CAD build for the part. Positions are in the model's coordinates, mm. Face numbers are marked on the shaded views. A direction names the side the tool comes from. Coordinates: 2 decimals unless noted, no trailing zeros. Order: outer loops, then holes, each group sorted by start corner. A loop starts at its lowest first (then second) coordinate and runs counter-clockwise, first axis right, second up. Notation, with made-up numbers: M -33,6.5 L 24,6.5 A28 cw 24,32.5 Z; hole C -34.75,-25.75 d11. An arc over 180 degrees is marked long. One line per item, written item: value.
from build123d import *

# Parameters (mm, degrees)
SKETCH_1_W                = 48.51
SKETCH_1_H                = 34
SKETCH_1_W_2              = 28.51
SKETCH_1_H_2              = 14
EXTRUDE_1_DEPTH           = 12.25
SKETCH_2_R                = 1.91
CUT_EXTRUDE_1_DEPTH       = 33.05257439
SKETCH_4_W                = 13
SKETCH_4_H                = 13.91
EXTRUDE_1_2_DEPTH         = 74.82
SKETCH_5_W                = 13.91
SKETCH_5_H                = 16.23
EXTRUDE_2_DEPTH           = 15
SKETCH_7_R                = 24.5
SKETCH_7_R_2              = 14.5
EXTRUDE_2_2_DEPTH         = 16.23
SKETCH_12_R               = 1.9
CUT_EXTRUDE_4_DEPTH       = 97.312124675
EXTRUDE_3_DEPTH           = 10
EXTRUDE_3_DEPTH_BACK      = 8
SKETCH_13_W               = 13.91
SKETCH_13_H               = 16.23
SKETCH_14_R               = 1.9
CUT_EXTRUDE_5_DEPTH       = 103.744583434
SKETCH_16_W               = 90.709398763
SKETCH_16_H               = 28.955068616
CUT_EXTRUDE_7_DEPTH       = 111.229011154
SKETCH_18_W               = 13
SKETCH_18_H               = 93.080932143
CUT_EXTRUDE_10_DEPTH      = 27
CUT_EXTRUDE_11_DEPTH      = 57
CUT_EXTRUDE_11_DEPTH_BACK = 27
SKETCH_17_W               = 20.23049449
SKETCH_17_H               = 80.723570055
SKETCH_21_W               = 15.09856282
SKETCH_21_H               = 42.5
EXTRUDE_6_DEPTH           = 10
SKETCH_22_R               = 4.005
CUT_EXTRUDE_12_DEPTH      = 24
SKETCH_23_W               = 15.09856282
SKETCH_23_H               = 4.587452919
CUT_EXTRUDE_13_DEPTH      = 85.439664289


with BuildPart() as part:
    # 草圖1 → Extrude 1 (new body)
    with BuildSketch(Plane(origin=(0, 0, 0), x_dir=(1, 0, 0), z_dir=(0, 1, 0))):
        Rectangle(SKETCH_1_W, SKETCH_1_H)
        Rectangle(SKETCH_1_W_2, SKETCH_1_H_2, mode=Mode.SUBTRACT)
    extrude(amount=EXTRUDE_1_DEPTH)

    # 草圖2 → 除料-伸長1 (cut, through all)
    with BuildSketch(Plane(origin=(0, 12.25, 0), x_dir=(1, 0, 0), z_dir=(0, 1, 0))):
        with Locations(Location((-19.255, 0, 0), (0, 0, 270))):
            Circle(SKETCH_2_R)
        with Locations(Location((19.255, 0, 0), (0, 0, 270))):
            Circle(SKETCH_2_R)
    extrude(amount=-CUT_EXTRUDE_1_DEPTH, mode=Mode.SUBTRACT)

    # 草圖4 → Extrude 1 2 (add)
    with BuildSketch(Plane.XZ):
        with Locations((17.755, 0)):
            Rectangle(SKETCH_4_W, SKETCH_4_H)
    extrude(amount=EXTRUDE_1_2_DEPTH)

    # 草圖5 → Extrude 2 (add)
    with BuildSketch(Plane.ZY.offset(-11.255)):
        with Locations((0, -66.705)):
            Rectangle(SKETCH_5_W, SKETCH_5_H)
    extrude(amount=EXTRUDE_2_DEPTH)

    # 草圖7 → Extrude 2 2 (add)
    with BuildSketch(Plane(origin=(3.626674765, -74.82, 0), x_dir=(1, 0, 0), z_dir=(0, -1, 0))):
        with Locations((-30.978154344, 0)):
            Circle(SKETCH_7_R)
        with Locations((-30.978154344, 0)):
            Circle(SKETCH_7_R_2, mode=Mode.SUBTRACT)
    extrude(amount=-EXTRUDE_2_2_DEPTH)

    # 草圖12 → 除料-伸長4 (cut, through all)
    with BuildSketch(Plane(origin=(0, 0, -6.955), x_dir=(-1, 0, 0), z_dir=(0, 0, -1))):
        with Locations((-3.856713649, -66.705)):
            Circle(SKETCH_12_R)
    extrude(amount=-CUT_EXTRUDE_4_DEPTH, mode=Mode.SUBTRACT)

    # 草圖13 → 填料-伸長3 (add, two sides: drawn at the far end of the back side and taken through both)
    with BuildSketch(Plane(origin=(-55, 0, 0), x_dir=(0, 0, -1), z_dir=(1, 0, 0)).offset(-EXTRUDE_3_DEPTH_BACK)):
        with Locations((0, -66.705)):
            Rectangle(SKETCH_13_W, SKETCH_13_H)
    extrude(amount=EXTRUDE_3_DEPTH + EXTRUDE_3_DEPTH_BACK)

    # 草圖14 → 除料-伸長5 (cut, through all)
    with BuildSketch(Plane(origin=(0, 0, -6.955), x_dir=(-1, 0, 0), z_dir=(0, 0, -1))):
        with Locations((56.908040017, -66.705)):
            Circle(SKETCH_14_R)
    extrude(amount=-CUT_EXTRUDE_5_DEPTH, mode=Mode.SUBTRACT)

    # 草圖16 → 除料-伸長7 (cut, through all)
    with BuildSketch(Plane(origin=(0, 12.25, 0), x_dir=(1, 0, 0), z_dir=(0, 1, 0))):
        with Locations((-17.645300619, -14.477534308)):
            Rectangle(SKETCH_16_W, SKETCH_16_H)
    extrude(amount=-CUT_EXTRUDE_7_DEPTH, mode=Mode.SUBTRACT)

    # 草圖18 → 除料-伸長10 (cut)
    with BuildSketch(Plane.XY):
        with Locations((17.755, -28.279533929)):
            Rectangle(SKETCH_18_W, SKETCH_18_H)
    extrude(amount=-CUT_EXTRUDE_10_DEPTH, mode=Mode.SUBTRACT)


with BuildPart() as cut_extrude_10_piece_1:
    # of the separate pieces the step leaves, piece 1, a body of its own (cut_extrude_10_pieces)
    add(part.part.solids().sort_by_distance((11.255, -58.59, -6.955))[0])

    # 草圖21 → 填料-伸長6 (add)
    with BuildSketch(Plane.XY.offset(-30)):
        with Locations((-27.29428141, -48.519427919)):
            Rectangle(SKETCH_21_W, SKETCH_21_H)
    extrude(amount=EXTRUDE_6_DEPTH)

    # 草圖22 → 除料-伸長12 (cut)
    with BuildSketch(Plane(origin=(0, -27.269427919, 0), x_dir=(1, 0, 0), z_dir=(0, 1, 0))):
        with Locations((-27.29428141, 20)):
            Circle(SKETCH_22_R)
    extrude(amount=-CUT_EXTRUDE_12_DEPTH, mode=Mode.SUBTRACT)

    # 草圖23 → 除料-伸長13 (cut, through all)
    with BuildSketch(Plane(origin=(0, -27.269427919, 0), x_dir=(1, 0, 0), z_dir=(0, 1, 0))):
        with Locations((-27.29428141, 27.706273541)):
            Rectangle(SKETCH_23_W, SKETCH_23_H)
    extrude(amount=-CUT_EXTRUDE_13_DEPTH, mode=Mode.SUBTRACT)


with BuildPart() as cut_extrude_10_piece_2:
    # of the separate pieces the step leaves, piece 2, a body of its own (cut_extrude_10_pieces)
    add(part.part.solids().sort_by_distance((-17.345, 0, 0))[0])

    # 草圖17 → 除料-伸長11 (cut, two sides: drawn at the far end of the back side and taken through both)
    with BuildSketch(Plane.ZY.offset(-11.255).offset(-CUT_EXTRUDE_11_DEPTH_BACK)):
        with Locations((-10.115247245, -18.228214973)):
            Rectangle(SKETCH_17_W, SKETCH_17_H)
    extrude(amount=CUT_EXTRUDE_11_DEPTH + CUT_EXTRUDE_11_DEPTH_BACK, mode=Mode.SUBTRACT)


solid = cut_extrude_10_piece_1.part
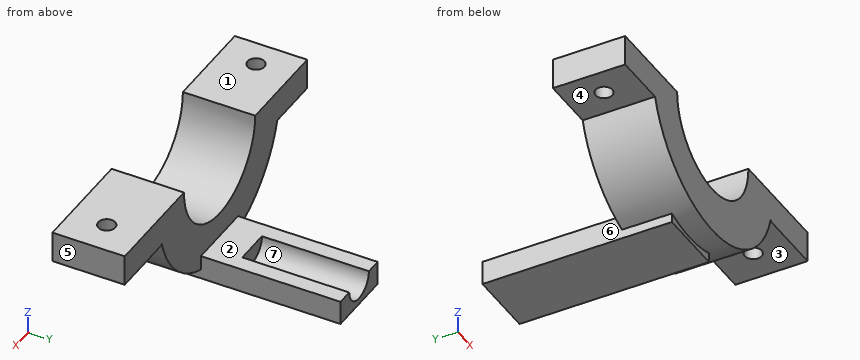
Q1. Slice it at B-B (y = -31). List the corners of the cut face in (x, z) (3 decimals).
Recorded:
outline: M -34.844,-25.413 L -19.745,-25.413 L -19.745,-20 L -23.289,-20 A4.005 cw -31.299,-20 L -34.844,-20 Z
Q2. Which spindle directions (+Z, -Z, +X, -X, +Y, -Y) get a long thin tool onto all of the face, cutting with end or side? Do the marked faces 1, 2 and 3. Say none if no direction does.
Recorded:
face 1: +Z, +X, -X, +Y, -Y
face 2: +Z, +X, -X, +Y
face 3: -Z, +X, +Y, -Y
Q3. Pin check, flat tips, straight feed: pin 1 Ø12 at (x, z) = (-40, -15.5) entering from +Y; pin 2 Ø2.5 at (x, y) = (-56.91, -66.7) entering from -Z; pin 3 Ø6 at (x, y) = (-6.5, -66) entering from +Z; pin 4 Ø4.5 at (y, z) = (-41.5, -23.5) entering from +X (3 decimals). Stop position of each tip, or through.
Recorded:
pin 1: stops at y = -58.59
pin 2: passes through
pin 3: stops at z = 0
pin 4: stops at x = -19.745
Q4. Slice it at D-D (x = -36.5). List the corners of the cut face in (y, z).
Recorded:
outline: M -74.82,-22.73 L -58.59,-22.73 L -58.59,-11.25 L -74.82,-11.25 Z
Q5. Slice it at A-A (x = -57.5). List the corners of the cut face in (y, z) (3 decimals), plus the area to 3 significant figures.
Recorded:
outline: M -74.82,-6.955 L -68.51,-6.955 L -68.51,0 L -74.82,0 Z; M -64.9,-6.955 L -58.59,-6.955 L -58.59,0 L -64.9,0 Z
area: 87.8 mm^2
Q6. Drill centre lines: line 1 along Y through (x, z) = (-20, -14.5); line 2 along X through (y, z) = (-54, -24) (3 decimals); line 3 along X through (y, z) = (-60, -8). Where is each one in solid material? Low to high.
Recorded:
line 1: y = -74.82 to -58.59
line 2: x = -34.844 to -19.745
line 3: x = -50.51 to -39.44, -15.26 to -4.19
Q7. Mould opens along X. For the marked faces 4, 5, 6 and 7 say: released by +X, released by -X, zero draft, split by the parting line, or undercut.
Recorded:
face 4: zero draft
face 5: released by +X
face 6: released by -X
face 7: undercut
Q8. Slice it at C-C (z = -8.75). List the corners of the cut face in (x, y), plus the area to 3 significant figures.
Recorded:
outline: M -50.24,-74.82 L -38.91,-74.82 L -38.91,-58.59 L -50.24,-58.59 Z; M -15.79,-74.82 L -4.47,-74.82 L -4.47,-58.59 L -15.79,-58.59 Z
area: 368 mm^2
